Build history of the part. All positions in model axes, mm. A direction names the side the tool comes from. Give positions to 0.01 mm unless a question says otherwise; leave off trailing zeros. Write each loop counter-clockwise with the first axis right and the second up, starting at its lowest first coordinate (ties: lowest second). Pieces come first, ordered by that corner, then holes. Notation, with made-up numbers: (32.5, -7.75) -> (77.5, -7.75) arc R12 cw to (77.5, 5.25) -> close; hole circle Ø1 at (62, 76.5). An arc over 180 degrees is marked (long way). Put each result on its own line as item: value. Start each with the question number.
Item 1: Drill centre lines: line 1 along Y through (x, z) = (21, 26.5); line 2 along Y through (x, z) = (11, 1.5); line 3 along Z through (x, y) = (5, 3.75). Where is each one in solid material? Low to high.
Item 2: Slice it at A-A, the plane y = 0. List the corners of the cut face in (x, z).
Item 3: Slice it at C-C, the plane z = 18.5. List the corners of the cut face in (x, y).
Item 4: Slice it at D-D, the plane y = -2.75. List the corners of the cut face in (x, z).
Item 5: Two-plate mould, pull along Y, no slides. Class faces 5 (the flat face through (0, 0, -9.7)), 6 (the flat face through (21, -7.5, 30)), 7 (the flat face through (21, 6.5, 30)), 8 (the flat face through (21, 7.5, 30)): pulls with the +Y half, pulls with the -Y half, needs draft (parallel to the pull), parting line crosses it, or undercut.
Item 6: Slice it at B-B, the plane x = 24. List the corners of the cut face in (y, z).
Item 7: Tool access for faces 1 (the flat face through (21, 11, 10.9)), 2 (the flat face through (2, 0, 13.9)), 3 (the flat face through (21, 11.3, 21)), 4 (the flat face through (21, -12, 13.9)): list every direction of +Z, -Z, +X, -X, +Y, -Y with a clear straight run to the whole face (end or side of a thin tool).
Item 8: Flat gauge pins, fed straight in: pin 1 Ø3.5 at (x, z) = (21.5, 18) entering from -Y; pin 2 Ø7 at (x, z) = (12.5, 4.5) entering from -Y; pin 3 Ø2.5 at (x, y) = (20, 11.5) entering from -Z. Where does each tip first touch, or does it go through?
```python
from build123d import *

# Parameters (mm, degrees)
F1_DEPTH = 13.9
F2_R     = 1.5
F3_DEPTH = 9.7
F4_W     = 11.5
F4_H     = 2.4
F5_DEPTH = 3
F6_W     = 11.5
F6_H     = 22.5
F7_DEPTH = 13.5
F8_R     = 0.75
F8_W     = 2
F8_H     = 1
F9_DEPTH = 5


with BuildPart() as f1:
    # F0 (on Top) → F1 (new body)
    with BuildSketch(Plane.XY):
        with BuildLine():
            Line((26.5, 10), (0, 10))
            ThreePointArc((0, 10), (-10, 0), (0, -10))
            Line((0, -10), (26.5, -10))
            Line((26.5, -10), (26.5, 10))
        make_face()
    extrude(amount=F1_DEPTH)

    # F2 (on face) → F3 (join)
    with BuildSketch(Plane(origin=(0, 0, 0), x_dir=(1, 0, 0), z_dir=(0, 0, -1))):
        Circle(F2_R)
    extrude(amount=F3_DEPTH)

    # F4 (on face) → F5 (join)
    with BuildSketch(Plane.XY.offset(13.9)):
        with Locations((20.75, 11.2)):
            Rectangle(F4_W, F4_H)
        with Locations((20.75, -11.2)):
            Rectangle(F4_W, F4_H)
    extrude(amount=-F5_DEPTH)

    # F6 (on face) → F7 (join)
    with BuildSketch(Plane.XY.offset(13.9)):
        with Locations((20.75, 0.05)):
            Rectangle(F6_W, F6_H)
    extrude(amount=F7_DEPTH)

    # F8 (on face) → F9 (join)
    with BuildSketch(Plane.XY.offset(27.4)):
        with Locations((20.75, 0)):
            Circle(F8_R)
        with Locations((20.75, 7)):
            Rectangle(F8_W, F8_H)
        with Locations((20.75, -7)):
            Rectangle(F8_W, F8_H)
    extrude(amount=F9_DEPTH)


solid = f1.part
```
Values follow:
1. line 1: -11.2 to 11.3
1. line 2: -10 to 10
1. line 3: 0 to 13.9
2. outline: (-10, 0) -> (-1.5, 0) -> (-1.5, -9.7) -> (1.5, -9.7) -> (1.5, 0) -> (26.5, 0) -> (26.5, 27.4) -> (21.5, 27.4) -> (21.5, 32.4) -> (20, 32.4) -> (20, 27.4) -> (15, 27.4) -> (15, 13.9) -> (-10, 13.9) -> close
3. outline: (15, -11.2) -> (26.5, -11.2) -> (26.5, 11.3) -> (15, 11.3) -> close
4. outline: (-9.61, 0) -> (26.5, 0) -> (26.5, 27.4) -> (15, 27.4) -> (15, 13.9) -> (-9.61, 13.9) -> close
5. face 5: needs draft
5. face 6: pulls with the -Y half
5. face 7: undercut
5. face 8: pulls with the +Y half
6. outline: (-12.4, 10.9) -> (-10, 10.9) -> (-10, 0) -> (10, 0) -> (10, 10.9) -> (12.4, 10.9) -> (12.4, 13.9) -> (11.3, 13.9) -> (11.3, 27.4) -> (-11.2, 27.4) -> (-11.2, 13.9) -> (-12.4, 13.9) -> close
7. face 1: -Z, +X, -X, +Y
7. face 2: +Z, -X, +Y, -Y
7. face 3: +Z, +X, -X, +Y
7. face 4: +Z, +X, -X, -Y
8. pin 1: y = -11.2
8. pin 2: y = -10
8. pin 3: z = 10.9
